The model under review builds one solid part; all positions refer to its coordinate system, in mm. A direction names the side the tool comes from. Coordinates: 2 decimals unless noted, no trailing zeros. Order: outer loops, then holes, each group sorted by start corner. A loop starts at its lowest first (then second) coordinate and runs counter-clockwise, first axis right, second up.
from build123d import *

# Parameters (mm, degrees)
BOSS_EXTRUDE1_DEPTH = 110
SKETCH2_R           = 2.6
CUT_EXTRUDE1_DEPTH  = 110
CUT_EXTRUDE2_START  = -7
CUT_EXTRUDE2_DEPTH  = 3
SKETCH4_R           = 2.6
CUT_EXTRUDE3_DEPTH  = 13


with BuildPart() as part:
    # Sketch1 → Boss-Extrude1 (new body)
    with BuildSketch(Plane.XY):
        Polygon((0, 0), (10, 0), (10, 13), (20, 13), (20, 20), (10, 20), (0, 20), align=None)
    extrude(amount=BOSS_EXTRUDE1_DEPTH)

    # Sketch2 → Cut-Extrude1 (cut)
    with BuildSketch(Plane(origin=(0, 20, 0), x_dir=(1, 0, 0), z_dir=(0, 1, 0))):
        with Locations((5, -21)):
            Circle(SKETCH2_R)
        with Locations((5, -89)):
            Circle(SKETCH2_R)
    extrude(amount=-CUT_EXTRUDE1_DEPTH, mode=Mode.SUBTRACT)

    # Sketch3 → Cut-Extrude2 (cut)
    with BuildSketch(Plane(origin=(0, 20, 0), x_dir=(1, 0, 0), z_dir=(0, 1, 0)).offset(CUT_EXTRUDE2_START)):
        Polygon((15, -50.438932873), (11.05, -52.719466437), (11.05, -57.280533563), (15, -59.561067127), (18.95, -57.280533563), (18.95, -52.719466437), align=None)
    extrude(amount=CUT_EXTRUDE2_DEPTH, mode=Mode.SUBTRACT)

    # Sketch4 → Cut-Extrude3 (cut)
    with BuildSketch(Plane.XZ.offset(-16)):
        with Locations((15, 55)):
            Circle(SKETCH4_R)
    extrude(amount=-CUT_EXTRUDE3_DEPTH, mode=Mode.SUBTRACT)


solid = part.part
(1) Insertion check: pin 1 Ø8.5 at (x, z) = (15, 55) entering from -Y; pin 2 Ø10.5 at (y, z) = (6.5, 76.5) entering from +X; pin 3 Ø1.5 at (x, z) = (16.5, 56) entering from +Y. Each pin has a flat end and moves straight along its axis. Give the tip position at first contact, or say it passes through.
(2) Consider section D-D (y = 3.25). Give the boundary of the cut face in (x, z), then the cut area to 3 significant figures.
(3) Consider section A-A (x = 5). Give the boundary of the cut face in (y, z).
(4) The part is to be moulded in two halves that separate along X. For faces 4 (the face through (19.4, 13, 54.2)), 5 (the face through (13.053, 14.479, 51.563)), 6 (the face through (20, 16, 54)), say which applies: +X half, -X half, draft (parallel to the pull), parting line (faces both ways), or undercut.
(5) Wall thickness on line 1 (Z direction, x = 5, y = 10.5); line 2 (X direction, y = 12.5, z = 21); line 3 (Z direction, x = 7.25, y = 1.25): over which ranges is each line inside the solid? List them lowest first.
(6) Consider section C-C (x = 16.25). Give the boundary of the cut face in (y, z).
(7) Consider section B-B (z = 89). Give the boundary of the cut face in (x, y), then the cut area to 3 significant figures.
(8) Tool access review of faces 1 (the face through (10, 6, 54)), 2 (the face through (17.003, 14.479, 51.595)), 3 (the face through (10, 20, 54)): name each direction out of +Z, -Z, +X, -X, +Y, -Y from which nothing blocks a thin tool from reaching the whole face with its end or side.
Findings:
1. pin 1: stops at y = 13
1. pin 2: stops at x = 10
1. pin 3: passes through
2. outline: (0, 0) - (10, 0) - (10, 110) - (0, 110) - close; hole circle Ø5.2 at (5, 21); hole circle Ø5.2 at (5, 89)
2. area: 1,060 mm2
3. outline: (0, 0) - (20, 0) - (20, 18.4) - (0, 18.4) - close; (0, 23.6) - (20, 23.6) - (20, 86.4) - (0, 86.4) - close; (0, 91.6) - (20, 91.6) - (20, 110) - (0, 110) - close
4. face 4: draft
4. face 5: undercut
4. face 6: +X half
5. line 1: z = 0 to 18.4, 23.6 to 86.4, 91.6 to 110
5. line 2: x = 0 to 2.4, 7.6 to 10
5. line 3: z = 0 to 19.7, 22.3 to 87.7, 90.3 to 110
6. outline: (13, 0) - (20, 0) - (20, 52.72) - (16, 52.72) - (16, 51.16) - (13, 51.16) - close; (13, 58.84) - (16, 58.84) - (16, 57.28) - (20, 57.28) - (20, 110) - (13, 110) - close
7. outline: (0, 0) - (2.4, 0) - (2.4, 20) - (0, 20) - close; (7.6, 0) - (10, 0) - (10, 13) - (20, 13) - (20, 20) - (7.6, 20) - close
7. area: 166 mm2
8. face 1: +Z, -Z, +X, -Y
8. face 2: -Y
8. face 3: +Z, -Z, +X, -X, +Y
